Can you work these out from the model? Positions are in its coordinate system, mm. A direction names the side the tool comes from. Coordinates: 2 decimals unless noted, no trailing zeros. Write each loop counter-clockwise with the first axis right and the second up, starting at its lowest first coordinate (ties: lowest second). Pieces come first, ordered by that corner, then holes. Notation, with made-up numbers: M 63.25,49.25 L 112.25,49.25 A21 ccw 112.25,85.25 Z; hole C 44,19 d5. An arc over 180 degrees is marked long. Answer as a JSON object with one key per item and string values. Group by question number.
from build123d import *

# Parameters (mm, degrees)
F0_W     = 25
F0_H     = 35
F1_DEPTH = 25
F2_W     = 20
F2_H     = 20
F3_DEPTH = 25
F5_D     = 5
F5_DEPTH = 20
F5_TIP   = 1.5021515476


with BuildPart() as f1:
    # F0 (on Top) → F1 (new body)
    with BuildSketch(Plane.XY):
        with Locations((12.5, 17.5)):
            Rectangle(F0_W, F0_H)
    extrude(amount=F1_DEPTH)

    # F2 (on face) → F3 (join)
    with BuildSketch(Plane.YZ.offset(25)):
        with Locations((25, 35)):
            Rectangle(F2_W, F2_H)
    extrude(amount=-F3_DEPTH)

    # F5
    with Locations(Plane.XY.offset(45)):
        with Locations((6.25, 25), (18.75, 25)):
            Hole(F5_D / 2, depth=F5_DEPTH)
            with Locations((0, 0, -(F5_DEPTH + F5_TIP / 2))):  # 118° drill point
                Cone(0, F5_D / 2, F5_TIP, mode=Mode.SUBTRACT)


solid = f1.part
Q1. If we section it at B-B on x = 14.5: List the corners of the cut face in (y, z) for me.
Q2. Will this pin go through, and if not, where does the flat tip stop? pin 1 (10 mm diameter, centred on x = 13, z = 31, fed in from -Y).
Q3. If we section it at A-A on z = 29.5: List the corners of the cut face in (x, y) for me, and give its area (3 significant figures).
Q4. We'd pull the mould along X, two halves only. Please class faces 1 (the flat face through (25, 21, 18)), 2 (the conical face through (5.816, 25.019, 23.759)), 3 (the flat face through (12, 18, 0)), 4 (the conical face through (19.15, 24.83, 23.76)): pulls with the +X half, pulls with the -X half, needs draft (parallel to the pull), parting line crosses it, or undercut.
Q5. On a 3-axis mill with a long thin cutter (end or side, diameter ignored), from which of +Z, -Z, +X, -X, +Y, -Y can I reach the whole of each face in a straight line? I mean faces 5 (the cylindrical face through (4.91, 27.11, 34.86)), 6 (the flat face through (0, 21, 18)), 7 (the flat face through (12, 8, 25)). Say none if no direction works.
Q6. Please list where these lines run through material, in increasing order: L1, parallel to X at y = 25, z = 33.5; L2, parallel to Y at x = 6.25, z = 35.5; L3, parallel to Y at x = 23.25, z = 29.5.
Q7. If we section it at C-C on y = 14: List the corners of the cut face in (x, z) for me, and give its area (3 significant figures).
Reply:
{
 "1": {"outline": "M 0,0 L 35,0 L 35,45 L 15,45 L 15,25 L 0,25 Z"},
 "2": {"pin 1": "y = 15"},
 "3": {"outline": "M 0,15 L 25,15 L 25,35 L 0,35 Z; hole C 6.25,25 d5; hole C 18.75,25 d5", "area": "461 mm^2"},
 "4": {"face 1": "pulls with the +X half", "face 2": "undercut", "face 3": "needs draft", "face 4": "undercut"},
 "5": {"face 5": "+Z", "face 6": "+Z, -Z, -X, +Y, -Y", "face 7": "+Z, +X, -X, -Y"},
 "6": {"L1": "0 to 3.75, 8.75 to 16.25, 21.25 to 25", "L2": "15 to 22.5, 27.5 to 35", "L3": "15 to 35"},
 "7": {"outline": "M 0,0 L 25,0 L 25,25 L 0,25 Z", "area": "625 mm^2"}
}
